The model under review builds one solid part; all positions refer to its coordinate system, in mm. Face numbers are marked on the shaded views. A direction names the side the tool comes from. Coordinates: 2 decimals unless noted, no trailing zeros. Order: outer loops, then holes, each group sorted by start corner. A loop starts at its lowest first (then second) coordinate and runs counter-clockwise, first axis right, second up. Notation, with made-up numbers: (29.25, 80) -> (86.25, 80) arc R32 ccw to (86.25, 112) -> close; hole circle Ø2 at (-26.5, 72). An arc over 180 degrees is marked (long way). Use CSV: the item, a comma, the result in double quotes. Start each with the question number.
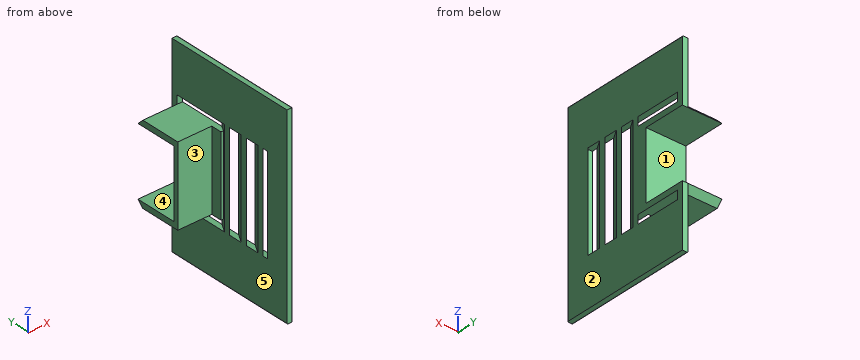
```python
from build123d import *

# Parameters (mm, degrees)
BOSS_EXTRU_3_DEPTH         = 5
ESQUISSE6_W                = 85.242430228
ESQUISSE6_H                = 5.217313119
R_P_TITION_START           = -42.621215114
R_P_TITION_LIN_AIRE1_DEPTH = 85.242430228
CONG_1_R                   = 1
BOSS_EXTRU_5_DEPTH         = 30


with BuildPart() as part:
    # Esquisse2 → Boss.-Extru.3 (new body)
    with BuildSketch(Plane(origin=(0, 0, 0), x_dir=(0, 0, -1), z_dir=(1, 0, 0))):
        Polygon((0, 25.151677918), (30, 25.151677918), (30, 62.151677918), (85, 62.151677918), (85, -55.200485129), (0, -55.200485129), (0, -35.567359792), (42.621215114, -35.567359792), (42.621215114, 57.151677918), (35, 57.151677918), (35, 12.151677918), (0, 12.151677918), align=None)
    boss_extru_3 = extrude(amount=BOSS_EXTRU_3_DEPTH)

    # Sym_trie1: Boss.-Extru.3 across plane
    add(boss_extru_3.mirror(Plane.XY))

    # Balayage5: sweep along a path in Esquisse5
    with BuildLine(Plane.XY.offset(-42.621215114)) as balayage5_path:
        Line((0, -30.703084538), (5, -22.249219394))
    # Esquisse6 → Balayage5 (sweep)
    with BuildSketch(Plane(origin=(0, 0, 0), x_dir=(0, 0, -1), z_dir=(1, 0, 0))):
        with Locations((0, -28.094427979)):
            Rectangle(ESQUISSE6_W, ESQUISSE6_H)
    sweep(path=balayage5_path.line)

    # R_p_tition lin_aire1: read off the stored shape, not the designer's step
    # R_p_tition lin_aire1 outline → R_p_tition lin_aire1 (add)
    with BuildSketch(Plane.XY.offset(R_P_TITION_START)):
        Polygon((5, -35.567359792), (5, -34.031906274), (4.091863017, -35.567359792), align=None)
        Polygon((0, -13.703084538), (5, -5.249219394), (5, -0.031906274), (0, -8.485771419), align=None)
        Polygon((0, 3.296915462), (5, 11.750780606), (5, 16.968093726), (0, 8.514228581), align=None)
    extrude(amount=R_P_TITION_LIN_AIRE1_DEPTH)

    # Cong_1
    cong_1_edges = [part.edges().sort_by_distance(p)[0] for p in [
        (0, 3.475596394, -85),
        (5, -55.200485129, 0),
        (5, 3.475596394, 85),
    ]]
    fillet(cong_1_edges, radius=CONG_1_R)

    # Esquisse8 → Boss.-Extru.5 (add)
    with BuildSketch(Plane.ZY):
        Polygon((-30, 62.151677918), (-30, 25.151677918), (30, 25.151677918), (30, 62.151677918), (35, 57.151677918), (35, 21.565276585), (-35, 21.565276585), (-35, 57.151677918), align=None)
    extrude(amount=BOSS_EXTRU_5_DEPTH)


solid = part.part
```
Q1. To check wall thickness, follow probe 1 along Z at (x, y) = (2, 32); probe 2 along Z at (x, y) = (2, 25); probe 3 along Z at (x, y) = (-17, 45). State the ranges of each line that lie inside material, in increasing order.
Q2. Add section A-A, the plane y = 38.5. State the section outline as (x, z) points, then the cut area to 3 significant figures.
Q3. Add section D-D, the plane z = 63. State the section outline as (x, y) points.
Q4. For the marked faces 1, 2 and 3, list the 3-axis set-ups (+Z, -Z, +X, -X, +Y, -Y) from which the entire face can be reached by the end or side of a thin tool; tool diameter is ignored.
Q5. Add section C-C, the plane x = -4. State the section outline as (y, z) points, then the cut area to 3 significant figures.
Q6. Clearance check with flat-ended pins moving along their axes: pin 1 Ø4 at (y, z) = (5.5, 67.5) entering from -X; pin 2 Ø1.5 at (x, y) = (-20.5, 39) entering from -Z; pin 3 Ø1.5 at (y, z) = (-29.5, 24.5) entering from +X; pin 4 Ø1 at (x, y) = (-2, -34) entering from +Z. State where each tip first meets the part, or that it passes through.
Q7. Draft analysis for pull direction Z (two halves, no side actions). For the marked faces 4 and 5, state which applies: +Z half, -Z half, draft (parallel to the pull), parting line (faces both ways), or undercut.
Q8. Add section B-B, the plane z = 22. State the section outline as (x, y) points, then the cut area to 3 significant figures.
Answer block:
1,probe 1,"z = -85 to -42.62, -35 to -30, 30 to 35, 42.62 to 85"
1,probe 2,"z = -85 to -42.62, -35 to 35, 42.62 to 85"
1,probe 3,"z = -35 to -30, 30 to 35"
2,outline,"(-30, -35) -> (5, -35) -> (5, -30) -> (-30, -30) -> close; (-30, 30) -> (5, 30) -> (5, 35) -> (-30, 35) -> close; (0, -84) arc R1 ccw to (1, -85) -> (5, -85) -> (5, -42.62) -> (0, -42.62) -> close; (0, 42.62) -> (5, 42.62) -> (5, 84) arc R1 ccw to (4, 85) -> (0, 85) -> close"
2,area,"773 mm²"
3,outline,"(0, -55.2) -> (4, -55.2) arc R1 ccw to (5, -54.2) -> (5, 62.15) -> (0, 62.15) -> close"
4,face 1,"+X, -X, +Y"
4,face 2,"+Z, -Z, +X, +Y, -Y"
4,face 3,"+Z, -Z, -X, -Y"
5,outline,"(21.57, -35) -> (57.15, -35) -> (62.15, -30) -> (25.15, -30) -> (25.15, 30) -> (62.15, 30) -> (57.15, 35) -> (21.57, 35) -> close"
5,area,"596 mm²"
6,pin 1,"stops at x = 0"
6,pin 2,"stops at z = -35"
6,pin 3,"stops at x = 1.16"
6,pin 4,"passes through"
7,face 4,"undercut"
7,face 5,"draft"
8,outline,"(-30, 21.57) -> (0, 21.57) -> (0, 12.15) -> (2.15, 12.15) -> (0, 8.51) -> (0, 3.3) -> (5, 11.75) -> (5, 25.15) -> (-30, 25.15) -> close; (0, -55.2) -> (4, -55.2) arc R1 ccw to (5, -54.2) -> (5, -34.03) -> (4.09, -35.57) -> (0, -35.57) -> close; (0, -30.7) -> (5, -22.25) -> (5, -17.03) -> (0, -25.49) -> close; (0, -13.7) -> (5, -5.25) -> (5, -0.03) -> (0, -8.49) -> close"
8,area,"343 mm²"
